Geometry check sheet. Reference: the model listing, model coordinates, mm. A direction names the side the tool comes from. Round coordinates to 2 decimals unless told otherwise and drop trailing zeros. Write each loop counter-clockwise with the first axis right and the second up, starting at its lowest first coordinate (ties: lowest second). Pieces come first, ordered by that corner, then holes. Notation, with made-up numbers: M -6.75,51.5 L 20.25,51.5 A16 cw 20.25,56.5 Z; hole C 32,-28 d5. An arc over 180 degrees is marked long. Put each result on its own line as item: value. Start each with the question number.
(1) Tool access check on faces 5 (the flat face through (12.7, 3, 60)), 6 (the flat face through (0, 0, 11)), 7 (the flat face through (-12.7, 3, 60)). Record the directions out of +Z, -Z, +X, -X, +Y, -Y that give a thin tool (end or side, any length) a straight path to the whole face; none if there is none.
(2) Section check A-A on y = 3. Count the separate pieces of the cut face and the enclosed holes in it, then the cut area to 3 significant figures.
(3) Gauge pin test, flat ends, axial feed: pin 1 (1.9 mm diameter, centred on y = 3, z = 52.5, fed in from +X); pin 2 (2 mm diameter, centred on x = 12.5, y = 0.5, fed in from +Z); pin 3 (1.5 mm diameter, centred on x = -10.5, y = 2.5, fed in from -Z). Record the tip position at first contact, or that the pin passes through.
(4) Section check B-B on z = 71. Record the cut outline in (x, y).
(5) Material ranges on probe 1 along X at (y, z) = (4, 0); probe 2 along Z at (x, y) = (-8, 3); probe 3 along Z at (x, y) = (-6, 1.5), recorded low to high.
(6) Section check C-C on x = 3. Record the cut outline in (y, z).
(7) Section check D-D on x = 26. Record the cut outline in (y, z), then the cut area to 3 significant figures.
(8) Mould release check, pull along X, two halves, no side actions. Record for faces 1 (the cylindrical face through (-14.93, 3.219, 33.755)), 2 (the cylindrical face through (-1.063, 3.219, 75.786)), 3 (the flat face through (0, 3, 81)), 4 (the cylindrical face through (-9.76, 3.13, 2.17)): pulls with the +X half, pulls with the -X half, needs draft (parallel to the pull), parting line crosses it, or undercut.
from build123d import *

# Parameters (mm, degrees)
BOSS_EXTRUDE1_DEPTH     = 6.35
SKETCH5_R               = 10
CUT_EXTRUDE1_DEPTH      = 88.694483863
F_3_8_CLEARANCE_HOLE1_D = 9.8044
FILLET1_R               = 25
M5_CLEARANCE_HOLE1_D    = 5.3
FILLET2_R               = 5


with BuildPart() as part:
    # Sketch1 → Boss-Extrude1 (new body)
    with BuildSketch(Plane(origin=(0, 0, 0), x_dir=(1, 0, 0), z_dir=(0, 1, 0))):
        with BuildLine():
            Line((-12.7, -81), (12.7, -81))
            Line((12.7, -81), (12.7, -30.458332193))
            ThreePointArc((12.7, -30.458332193), (0, 33), (-12.7, -30.458332193))
            Line((-12.7, -30.458332193), (-12.7, -81))
        make_face()
    extrude(amount=BOSS_EXTRUDE1_DEPTH)

    # Sketch5 → Cut-Extrude1 (cut, through all)
    with BuildSketch(Plane.XZ):
        with Locations(Location((0, 0, 0), (0, 0, 270))):
            Circle(SKETCH5_R)
    extrude(amount=-CUT_EXTRUDE1_DEPTH, mode=Mode.SUBTRACT)

    # 3/8 Clearance Hole1 (through all)
    with Locations(Plane(origin=(0, 0, 0), x_dir=(-1, 0, 0), z_dir=(0, -1, 0))):
        with Locations((0, -46), (0, -71)):
            Hole(F_3_8_CLEARANCE_HOLE1_D / 2)

    # Fillet1
    fillet1_edges = [part.edges().sort_by_distance(p)[0] for p in [
        (-12.7, 3.175, 30.458332193),
        (12.7, 3.175, 30.458332193),
    ]]
    fillet(fillet1_edges, radius=FILLET1_R)

    # M5 Clearance Hole1 (through all)
    with Locations(Plane(origin=(0, 0, 0), x_dir=(-1, 0, 0), z_dir=(0, -1, 0))):
        with Locations((8, 24), (-12, 24), (-26, 10), (-26, -10), (-12, -24), (8, -24)):
            Hole(M5_CLEARANCE_HOLE1_D / 2)

    # Fillet2
    fillet2_edges = [part.edges().sort_by_distance(p)[0] for p in [
        (12.7, 3.175, 81),
        (-12.7, 3.175, 81),
    ]]
    fillet(fillet2_edges, radius=FILLET2_R)


solid = part.part
Answers follow:
1. face 5: +Z, +X, +Y, -Y
1. face 6: +Z, -Z, +X, -X, -Y
1. face 7: +Z, -X, +Y, -Y
2. separate pieces: 1
2. enclosed holes: 9
2. area: 4,100 mm^2
3. pin 1: stops at x = 12.7
3. pin 2: stops at z = 79.25
3. pin 3: stops at z = -31.53
4. outline: M -12.7,0 L -4.9,0 L -4.9,6.35 L -12.7,6.35 Z; M 4.9,0 L 12.7,0 L 12.7,6.35 L 4.9,6.35 Z
5. probe 1: x = -33 to -10, 10 to 33
5. probe 2: z = -32.02 to -26.65, -21.35 to -6, 6 to 21.35, 26.65 to 80.99
5. probe 3: z = -32.45 to -25.74, -22.26 to -8, 8 to 22.26, 25.74 to 81
6. outline: M 0,-32.86 L 6.35,-32.86 L 6.35,-9.54 L 0,-9.54 Z; M 0,9.54 L 6.35,9.54 L 6.35,42.12 L 0,42.12 Z; M 0,49.88 L 6.35,49.88 L 6.35,67.12 L 0,67.12 Z; M 0,74.88 L 6.35,74.88 L 6.35,81 L 0,81 Z
7. outline: M 0,-20.32 L 6.35,-20.32 L 6.35,-12.65 L 0,-12.65 Z; M 0,-7.35 L 6.35,-7.35 L 6.35,7.35 L 0,7.35 Z; M 0,12.65 L 6.35,12.65 L 6.35,20.32 L 0,20.32 Z
7. area: 191 mm^2
8. face 1: pulls with the -X half
8. face 2: undercut
8. face 3: needs draft
8. face 4: undercut
